The listing builds one solid part. Answer for the finished solid, in the listing's coordinates (mm). A direction names the side the tool comes from. Round coordinates to 2 decimals unless told otherwise and drop trailing zeros. Write each loop counter-clockwise with the first axis right and the second up, starting at its lowest first coordinate (ties: lowest second). Pieces come first, ordered by that corner, then holes. Notation, with made-up numbers: M -12.5,47 L 26.5,47 A21 ccw 26.5,79 Z; hole C 71,41.25 d11. An arc over 180 degrees is marked long. Answer as CSV lines item,"result". Start each with the question number.
from build123d import *

# Parameters (mm, degrees)
F0_W     = 20
F0_H     = 20
F1_DEPTH = 20
F2_T     = -2.5
F3_SIZE  = 2


with BuildPart() as f1:
    # F0 (on Front) → F1 (new body)
    with BuildSketch(Plane.XZ):
        with Locations((-10, 10)):
            Rectangle(F0_W, F0_H)
    extrude(amount=F1_DEPTH)

    # F2
    f2_openings = [f1.faces().sort_by_distance(p)[0] for p in [
        (-10, -10, 20),
    ]]
    offset(amount=F2_T, openings=f2_openings)

    # F3
    f3_edges = [f1.edges().sort_by_distance(p)[0] for p in [
        (-17.5, -10, 20),
        (-10, -2.5, 20),
        (-2.5, -10, 20),
        (-10, -17.5, 20),
    ]]
    chamfer(f3_edges, length=F3_SIZE)


solid = f1.part
Q1. Find section B-B (y = -9.5). Determine the outline of the cut face in (x, z), plus the area to 4 significant figures.
Q2. The mould has two halves that part along Y. Classify faces 1 (the face through (-10.1, -18.5, 19)), 2 (the face through (-10, 0, 10)), 3 (the face through (-10, -20, 10)), 4 (the face through (-20, -10, 10)): +Y half, -Y half, draft (parallel to the pull), parting line (faces both ways), or undercut.
Q3. Find section A-A (z = 13.5). Determine the outline of the cut face in (x, y).
Q4. Straight lines are drawn through the part: L1, parallel to Y at x = -3.5, z = 11; L2, parallel to Z at x = -3, y = -4.5. For each, find the intervals that lie inside material, in ascending order.
Q5. For faces 5 (the face through (-19.7, -10, 20)), 6 (the face through (-17.5, -10, 10)), determine the directions among +Z, -Z, +X, -X, +Y, -Y from which every point of the face is accessible in a straight line to the end or side of a thin tool.
Q6. Each of these flat-tipped pins is pushed along its axis until it touches: P1, Ø12, axis at x = -8, y = -10.5, coming from the +Z side; P2, Ø2, axis at x = -11.5, y = -8, coming from the +Z side. Where does it stop, or does it pass through?
Q7. Find section C-C (x = -1.5). Determine the outline of the cut face in (y, z).
Reported:
1,outline,"M -20,0 L 0,0 L 0,20 L -0.5,20 L -2.5,18 L -2.5,2.5 L -17.5,2.5 L -17.5,18 L -19.5,20 L -20,20 Z"
1,area,"133.5 mm2"
2,face 1,"undercut"
2,face 2,"+Y half"
2,face 3,"-Y half"
2,face 4,"draft"
3,outline,"M -20,-20 L 0,-20 L 0,0 L -20,0 Z; hole M -17.5,-17.5 L -2.5,-17.5 L -2.5,-2.5 L -17.5,-2.5 Z"
4,L1,"y = -20 to -17.5, -2.5 to 0"
4,L2,"z = 0 to 2.5"
5,face 5,"+Z, +X, -X, +Y, -Y"
5,face 6,"+Z"
6,P1,"stops at z = 18.5"
6,P2,"stops at z = 2.5"
7,outline,"M -20,0 L 0,0 L 0,20 L -0.5,20 L -1.5,19 L -18.5,19 L -19.5,20 L -20,20 Z"
